Input: dimensioned drawing with shaded views. Units: mm. Origin: part minimum x, y, z. A direction names the side the tool comes from. Round coordinates to 2 decimals unless told otherwise and drop trailing zeros. Write each loop counter-clockwise with the first axis right and the second up, starting at its lowest first coordinate (ties: lowest second). Pieces come first, ordered by that corner, then holes. Notation, with made-up numbers: (47, 36) -> (94, 36) arc R21 ccw to (94, 72) -> close; hole circle Ø4 at (-27, 21). An arc over 180 degrees is marked (long way). Return JSON: item names as keys, results as strings. Group by question number.
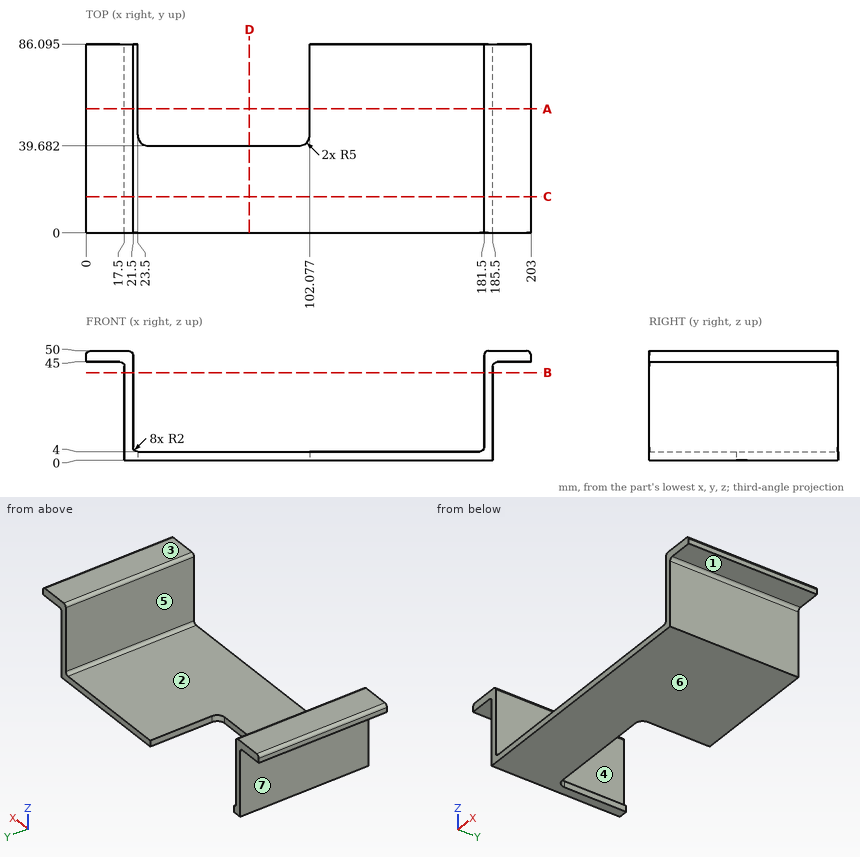
Item 1: Cut plane B-B on z = 40. Output: boundary loops of the cut face in (x, y) (3 decimals).
Item 2: Cut plane A-A on y = 56.5. Output: boundary loops of the cut face in (x, z), and give its area (3 significant figures).
Item 3: First-contact query: pin 1 Ø1.2 at (y, z) = (60, 2.5) entering from +X; pin 2 Ø1.2 at (y, z) = (74.5, 2) entering from -X; pin 3 Ø4.5 at (x, z) = (59, 1.5) entering from +Y. Flat tips, straight axial feed; report the tip coordinate or a pass-through.
Item 4: Cut plane D-D on x = 74.5. Output: boundary loops of the cut face in (y, z), and give its area (3 significant figures).
Item 5: Material intervals for probe 1 along X at (y, z) = (16, 39); probe 2 along X at (y, z) = (30.5, 47); probe 3 along Z at (x, y) = (138, 68.5), sorted ascending.
Item 6: Set-up query: the marked faces 1, 2 and 3. Return all of +Z, -Z, +X, -X, +Y, -Y with unobstructed straight access to the full face (end or side cutting, diameter ignored); none if empty.
Item 7: Cut plane C-C on y = 16.5. Output: boundary loops of the cut face in (x, z), and give its area (4 significant figures).
Item 8: Pull-direction query (X, two-part tool) for the marked faces 4, 5, 6 and 7; classes: +X half, -X half, draft (parallel to the pull), parting line (faces both ways), or undercut.
Here are the results:
{
 "1": {"outline": "(17.5, 0) -> (21.5, 0) -> (21.5, 86.095) -> (17.5, 86.095) -> close; (181.5, 0) -> (185.5, 0) -> (185.5, 86.095) -> (181.5, 86.095) -> close"},
 "2": {"outline": "(0, 45) -> (15.5, 45) arc R2 cw to (17.5, 43) -> (17.5, 0) -> (23.5, 0) -> (23.5, 4) arc R2 cw to (21.5, 6) -> (21.5, 48) arc R2 ccw to (19.5, 50) -> (2, 50) arc R2 ccw to (0, 48) -> close; (102.08, 0) -> (185.5, 0) -> (185.5, 43) arc R2 cw to (187.5, 45) -> (203, 45) -> (203, 48) arc R2 ccw to (201, 50) -> (183.5, 50) arc R2 ccw to (181.5, 48) -> (181.5, 6) arc R2 cw to (179.5, 4) -> (102.08, 4) -> close", "area": "901 mm^2"},
 "3": {"pin 1": "stops at x = 185.5", "pin 2": "stops at x = 17.5", "pin 3": "stops at y = 39.68"},
 "4": {"outline": "(0, 0) -> (39.68, 0) -> (39.68, 4) -> (0, 4) -> close", "area": "159 mm^2"},
 "5": {"probe 1": "x = 17.5 to 21.5, 181.5 to 185.5", "probe 2": "x = 0 to 21.5, 181.5 to 203", "probe 3": "z = 0 to 4"},
 "6": {"face 1": "-Z, +X, +Y, -Y", "face 2": "+Z, +Y, -Y", "face 3": "+Z, +X, -X, +Y, -Y"},
 "7": {"outline": "(0, 45) -> (15.5, 45) arc R2 cw to (17.5, 43) -> (17.5, 0) -> (185.5, 0) -> (185.5, 43) arc R2 cw to (187.5, 45) -> (203, 45) -> (203, 48) arc R2 ccw to (201, 50) -> (183.5, 50) arc R2 ccw to (181.5, 48) -> (181.5, 6) arc R2 cw to (179.5, 4) -> (23.5, 4) arc R2 cw to (21.5, 6) -> (21.5, 48) arc R2 ccw to (19.5, 50) -> (2, 50) arc R2 ccw to (0, 48) -> close", "area": "1,215 mm^2"},
 "8": {"face 4": "undercut", "face 5": "undercut", "face 6": "draft", "face 7": "-X half"}
}
